Geometry: final body of the model. Coordinates: model frame, mm. Face numbers are marked on the shaded views. A direction names the side the tool comes from. Give positions to 0.01 mm unless a question says otherwise; leave off trailing zeros. Order: outer loops, then holes, each group sorted by start corner. A loop starts at its lowest first (then second) coordinate and runs counter-clockwise, first axis right, second up. Notation, with made-up numbers: (-38, 76.5) -> (14, 76.5) arc R32 cw to (14, 109.5) -> close; hole circle Ø5 at (57, -34). An arc over 180 degrees is marked (long way). Write item = value, one per line.
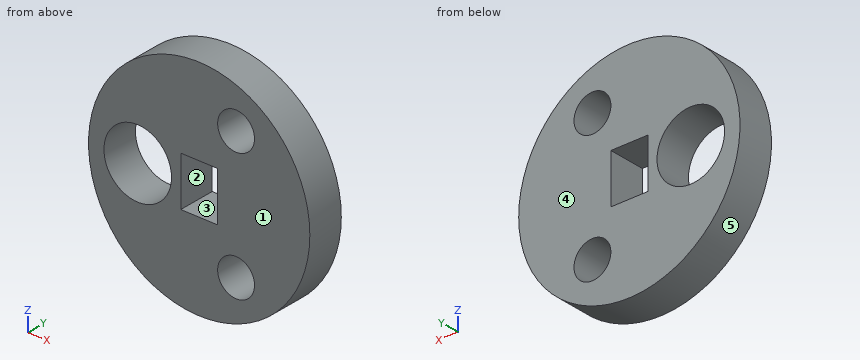
```python
from build123d import *

# Parameters (mm, degrees)
SKETCH1_R           = 9
SKETCH1_R_2         = 2.75
SKETCH1_R_3         = 1.5
SKETCH1_W           = 3
SKETCH1_H           = 4
BOSS_EXTRUDE1_DEPTH = 3


with BuildPart() as part:
    # Sketch1 → Boss-Extrude1 (new body)
    with BuildSketch(Plane(origin=(0, 0, 0), x_dir=(1, 0, 0), z_dir=(0, 1, 0))):
        Circle(SKETCH1_R)
        with Locations((-5, 0.000835232)):
            Circle(SKETCH1_R_2, mode=Mode.SUBTRACT)
        with Locations((2.999131959, -5.19665349)):
            Circle(SKETCH1_R_3, mode=Mode.SUBTRACT)
        with Locations((3.000867957, 5.195651211)):
            Circle(SKETCH1_R_3, mode=Mode.SUBTRACT)
        Rectangle(SKETCH1_W, SKETCH1_H, mode=Mode.SUBTRACT)
    extrude(amount=BOSS_EXTRUDE1_DEPTH)


solid = part.part
```
1) Section query A-A (x = 0). Output: boundary loops of the cut face in (y, z).
Check sheet entries:
outline = (0, -9) -> (3, -9) -> (3, -2) -> (0, -2) -> close; (0, 2) -> (3, 2) -> (3, 9) -> (0, 9) -> close
2) Line query: line 1 (Z direction, x = 4, y = 1.8); line 2 (X direction, y = 1.1, z = 0.5); line 3 (X direction, y = 0.35, z = 1.25). Output: solid intervals per line, ascending. Write a range as from..to.
Check sheet entries:
line_1 = -8.06..-6.31, -4.08..4.08, 6.31..8.06
line_2 = -8.99..-7.7, -2.3..-1.5, 1.5..8.99
line_3 = -8.91..-7.45, -2.55..-1.5, 1.5..8.91
3) Reachability of the marked faces 1 and 2 from +Z, -Z, +X, -X, +Y, -Y: full face, straight path, thin tool, end or side. Return the list, or none.
Check sheet entries:
face_1 = +Z, -Z, +X, -X, -Y
face_2 = +Y, -Y
4) First-contact query: P1, Ø0.9, axis at y = 1, z = 1, coming from the +X side. Flat tip, straight axial feed; report the tip coordinate or a pass-through.
Check sheet entries:
P1 = 8.98
5) Section query D-D (y = 0.7). Output: boundary loops of the cut face in (x, z), plus the area to 3 significant figures.
Check sheet entries:
outline = circle Ø18 at (0, 0); hole circle Ø5.5 at (-5, 0); hole (-1.5, -2) -> (1.5, -2) -> (1.5, 2) -> (-1.5, 2) -> close; hole circle Ø3 at (3, -5.2); hole circle Ø3 at (3, 5.2)
area = 205 mm²
6) Mould query, pull axis Z, two halves, no side actions, for the marked faces 3, 4 and 5. Classes: +Z half, -Z half, draft (parallel to the pull), parting line (faces both ways), or undercut.
Check sheet entries:
face_3 = undercut
face_4 = draft
face_5 = parting line
7) Section query B-B (z = 4.25). Output: boundary loops of the cut face in (x, y).
Check sheet entries:
outline = (-7.93, 0) -> (1.84, 0) -> (1.84, 3) -> (-7.93, 3) -> close; (4.16, 0) -> (7.93, 0) -> (7.93, 3) -> (4.16, 3) -> close
8) Section query C-C (z = -0.25). Output: boundary loops of the cut face in (x, y), plus the area to 3 significant figures.
Check sheet entries:
outline = (-9, 0) -> (-7.74, 0) -> (-7.74, 3) -> (-9, 3) -> close; (-2.26, 0) -> (-1.5, 0) -> (-1.5, 3) -> (-2.26, 3) -> close; (1.5, 0) -> (9, 0) -> (9, 3) -> (1.5, 3) -> close
area = 28.5 mm²
